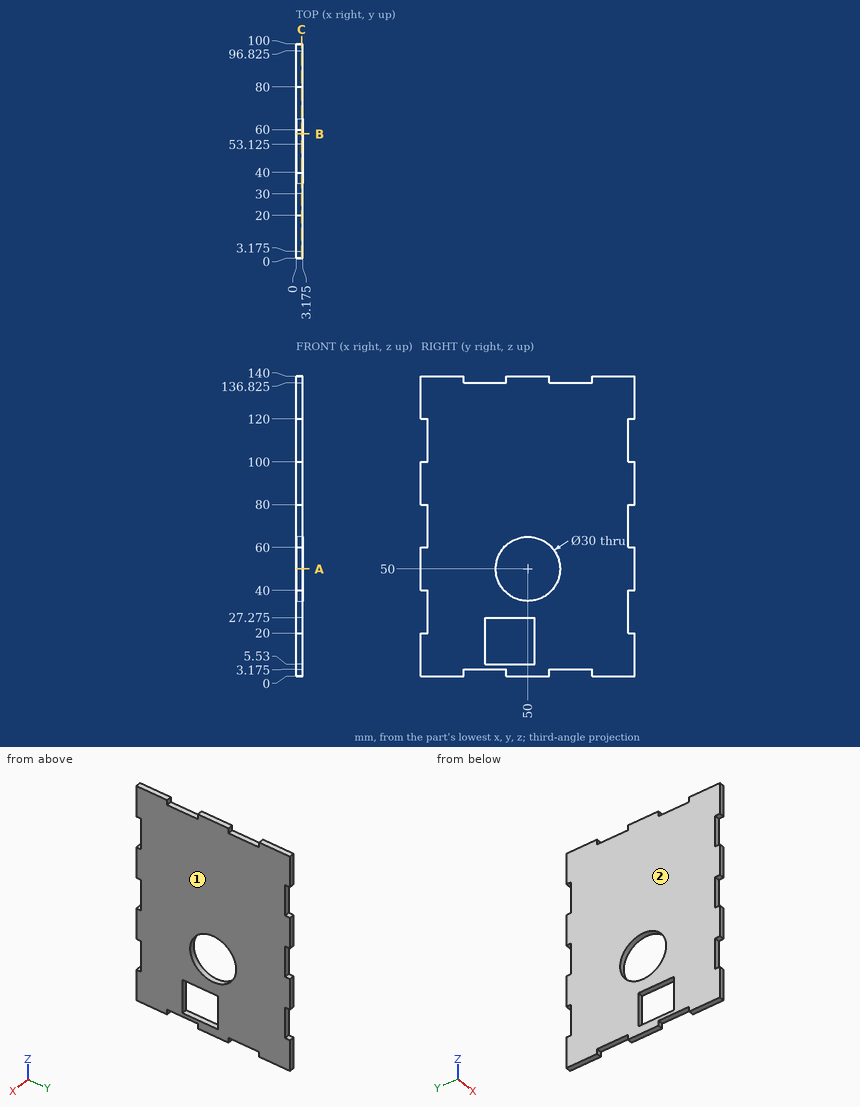
Check sheet for the drawn part. Datum: minimum x, y, z corner. Units: mm. Coordinates: 2 decimals unless noted, no trailing zeros. Order: outer loops, then holes, each group sorted by start corner. A loop starts at its lowest first (then second) coordinate and runs counter-clockwise, first axis right, second up. Notation, with made-up numbers: (4, 80.5) -> (23, 80.5) arc R20 ccw to (23, 95.5) -> close; hole circle Ø8 at (-27.5, 44.5). An arc over 180 degrees is marked (long way). Use a Markdown table: item, result. Add a question column.
1. Mould release check, pull along X, two halves, no side actions. Record for the marked faces 1 and 2: pulls with the +X half, pulls with the -X half, needs draft (parallel to the pull), parting line crosses it, or undercut.
2. Cross-section at B-B (y = 58). Enter the section's corners in (x, z) (3 decimals), and give its area (3 significant figures).
3. Cross-section at A-A (z = 50). Enter the section's corners in (x, y) (3 decimals).
4. Cross-section at C-C (x = 2.65). Give the number of separate pieces and of enclosed holes in the cut face, and give its area (3 significant figures).
5. Go/stop test with flat-tipped pins: pin 1 Ø1.6 at (x, z) = (1, 137.5) entering from -Y; pin 2 Ø1 at (x, y) = (1.5, 67) entering from -Z (3 decimals). Record where each tip stops, or that it passes through.
6. Material ranges on L1, parallel to Z at x = 2.3, y = 51 (3 decimals); L2, parallel to Y at x = 1.55, z = 50; L3, parallel to Z at x = 3, y = 47.5 (3 decimals), recorded low to high.
Filled sheet:
| question | item | result |
|---|---|---|
| 1 | face 1 | pulls with the +X half |
| 1 | face 2 | pulls with the -X half |
| 2 | outline | (0, 0) -> (3.175, 0) -> (3.175, 37.311) -> (0, 37.311) -> close; (0, 62.689) -> (3.175, 62.689) -> (3.175, 140) -> (0, 140) -> close |
| 2 | area | 364 mm2 |
| 3 | outline | (0, 0) -> (3.175, 0) -> (3.175, 35) -> (0, 35) -> close; (0, 65) -> (3.175, 65) -> (3.175, 100) -> (0, 100) -> close |
| 4 | separate pieces | 1 |
| 4 | enclosed holes | 2 |
| 4 | area | 12,200 mm2 |
| 5 | pin 1 | y = 0 |
| 5 | pin 2 | z = 3.175 |
| 6 | L1 | 0 to 5.53, 27.275 to 35.033, 64.967 to 140 |
| 6 | L2 | 0 to 35, 65 to 100 |
| 6 | L3 | 0 to 5.53, 27.275 to 35.21, 64.79 to 140 |
